from build123d import *

# Parameters (mm, degrees)
BOSS_EXTRUDE1_START = -85
SKETCH1_W           = 80
SKETCH1_H           = 12
BOSS_EXTRUDE1_DEPTH = 170
BOSS_EXTRUDE2_START = -83
SKETCH2_W           = 76
SKETCH2_H           = 14
BOSS_EXTRUDE2_DEPTH = 166
BOSS_EXTRUDE3_START = -82.6
SKETCH3_W           = 75.2
SKETCH3_H           = 16.5
BOSS_EXTRUDE3_DEPTH = 165.2
BOSS_EXTRUDE4_START = -80.6
SKETCH4_W           = 71.2
SKETCH4_H           = 17
BOSS_EXTRUDE4_DEPTH = 161.2
BOSS_EXTRUDE5_START = 50
SKETCH5_W           = 30
SKETCH5_H           = 10
BOSS_EXTRUDE5_DEPTH = 24
BOSS_EXTRUDE6_START = -74
SKETCH6_W           = 8
SKETCH6_H           = 10
BOSS_EXTRUDE6_DEPTH = 8
BOSS_EXTRUDE7_START = -45
SKETCH7_R           = 1.1
BOSS_EXTRUDE7_DEPTH = 90
BOSS_EXTRUDE8_START = -45
SKETCH8_R           = 1.1
BOSS_EXTRUDE8_DEPTH = 90


with BuildPart() as part:
    # Sketch1 → Boss-Extrude1 (new body)
    with BuildSketch(Plane.XY.offset(BOSS_EXTRUDE1_START)):
        with Locations((0, 40)):
            Rectangle(SKETCH1_W, SKETCH1_H)
    extrude(amount=BOSS_EXTRUDE1_DEPTH)


with BuildPart() as body_2:
    # Sketch2 → Boss-Extrude2 (new body)
    with BuildSketch(Plane.XY.offset(BOSS_EXTRUDE2_START)):
        with Locations((0, 37)):
            Rectangle(SKETCH2_W, SKETCH2_H)
    extrude(amount=BOSS_EXTRUDE2_DEPTH)


with BuildPart() as part_1:
    add(part.part)

    # Combine1: cut body 2
    add(body_2.part, mode=Mode.SUBTRACT)

    # Sketch3 → Boss-Extrude3 (add)
    with BuildSketch(Plane.XY.offset(BOSS_EXTRUDE3_START)):
        with Locations((0, 36.25)):
            Rectangle(SKETCH3_W, SKETCH3_H)
    extrude(amount=BOSS_EXTRUDE3_DEPTH)


with BuildPart() as body_2_2:
    # Sketch4 → Boss-Extrude4 (new body)
    with BuildSketch(Plane.XY.offset(BOSS_EXTRUDE4_START)):
        with Locations((0, 35.5)):
            Rectangle(SKETCH4_W, SKETCH4_H)
    extrude(amount=BOSS_EXTRUDE4_DEPTH)


with BuildPart() as part_2:
    add(part_1.part)

    # Combine2: cut body 2 2
    add(body_2_2.part, mode=Mode.SUBTRACT)


with BuildPart() as body_2_3:
    # Sketch5 → Boss-Extrude5 (new body)
    with BuildSketch(Plane.XY.offset(BOSS_EXTRUDE5_START)):
        with Locations((0, 45)):
            Rectangle(SKETCH5_W, SKETCH5_H)
    extrude(amount=BOSS_EXTRUDE5_DEPTH)


with BuildPart() as part_3:
    add(part_2.part)

    # Combine3: cut body 2 3
    add(body_2_3.part, mode=Mode.SUBTRACT)


with BuildPart() as body_2_4:
    # Sketch6 → Boss-Extrude6 (new body)
    with BuildSketch(Plane.XY.offset(BOSS_EXTRUDE6_START)):
        with Locations((0, 45)):
            Rectangle(SKETCH6_W, SKETCH6_H)
    extrude(amount=BOSS_EXTRUDE6_DEPTH)


with BuildPart() as part_4:
    add(part_3.part)

    # Combine4: cut body 2 4
    add(body_2_4.part, mode=Mode.SUBTRACT)


with BuildPart() as body_2_5:
    # Sketch7 → Boss-Extrude7 (new body)
    with BuildSketch(Plane(origin=(0, 0, 0), x_dir=(0, 0, -1), z_dir=(1, 0, 0)).offset(BOSS_EXTRUDE7_START)):
        with Locations(Location((30, 30, 0), (0, 0, 180))):
            Circle(SKETCH7_R)
    extrude(amount=BOSS_EXTRUDE7_DEPTH)


with BuildPart() as part_5:
    add(part_4.part)

    # Combine5: cut body 2 5
    add(body_2_5.part, mode=Mode.SUBTRACT)


with BuildPart() as body_2_6:
    # Sketch8 → Boss-Extrude8 (new body)
    with BuildSketch(Plane(origin=(0, 0, 0), x_dir=(0, 0, -1), z_dir=(1, 0, 0)).offset(BOSS_EXTRUDE8_START)):
        with Locations(Location((-30, 30, 0), (0, 0, 180))):
            Circle(SKETCH8_R)
    extrude(amount=BOSS_EXTRUDE8_DEPTH)


with BuildPart() as part_6:
    add(part_5.part)

    # Combine6: cut body 2 6
    add(body_2_6.part, mode=Mode.SUBTRACT)


solid = part_6.part
Source: CAD feature listing. Evaluate the final solid. Frame: model axes, mm. A direction names the side the tool comes from. Round coordinates to 2 decimals unless told otherwise and drop trailing zeros. Write each loop counter-clockwise with the first axis right and the second up, starting at its lowest first coordinate (ties: lowest second). Pieces come first, ordered by that corner, then holes. Notation, with made-up numbers: (-23.75, -25.75) - (22.25, -25.75) arc R14 ccw to (22.25, -13.75) - close; hole circle Ø2 at (87.25, 81.5). An arc over 180 degrees is marked (long way). Use CSV: the item, a comma, the result in double quotes. Start each with the question number.
(1) Cut plane B-B, the plane x = 28. Return loops of the section in (y, z).
(2) Cut plane C-C, the plane z = 33. Return loops of the section in (x, y), and give its area (3 significant figures).
(3) First-contact query: pin 1 Ø12 at (x, z) = (-2, -61.5) entering from -Y; pin 2 Ø8 at (x, y) = (17.5, 33) entering from +Z. Flat tips, straight axial feed; report the tip coordinate or a pass-through.
(4) Material intervals for probe 1 along X at (y, z) = (40, 32); probe 2 along Z at (x, y) = (-31, 41.5); probe 3 along Z at (x, y) = (36, 36), sorted ascending. Write a range as [from, to].
(5) Mould query, pull axis Z, two halves, no side actions, for faces 3 (the face through (-1, 36, 82.6)), 4 (the face through (-1, 40, 85)), 5 (the face through (36, 28, 0)). Classes: pulls with the +Z half, pulls with the -Z half, needs draft (parallel to the pull), parting line crosses it, or undercut.
(6) Cut plane A-A, the plane y = 41.5. Return loops of the section in (x, z), and give its area (3 significant figures).
(7) Set-up query: faces 1 (the face through (0, 36, 80.6)), 2 (the face through (-40, 40, -1)). Return all of +Z, -Z, +X, -X, +Y, -Y with unobstructed straight access to the full face (end or side cutting, diameter ignored); none if empty.
Geometry says:
1,outline,"(28, -82.6) - (44, -82.6) - (44, -83) - (34, -83) - (34, -85) - (46, -85) - (46, 85) - (34, 85) - (34, 83) - (44, 83) - (44, 82.6) - (28, 82.6) - (28, 80.6) - (44, 80.6) - (44, -80.6) - (28, -80.6) - close"
2,outline,"(-40, 34) - (-38, 34) - (-38, 44) - (-37.6, 44) - (-37.6, 28) - (-35.6, 28) - (-35.6, 44) - (35.6, 44) - (35.6, 28) - (37.6, 28) - (37.6, 44) - (38, 44) - (38, 34) - (40, 34) - (40, 46) - (-40, 46) - close"
2,area,"264 mm²"
3,pin 1,"y = 44"
3,pin 2,"z = 85"
4,probe 1,"[-40, -38], [-37.6, -35.6], [35.6, 37.6], [38, 40]"
4,probe 2,"[-85, -83], [-82.6, -80.6], [80.6, 82.6], [83, 85]"
4,probe 3,"[-85, -83], [-82.6, 82.6], [83, 85]"
5,face 3,"undercut"
5,face 4,"pulls with the +Z half"
5,face 5,"needs draft"
6,outline,"(-40, -85) - (40, -85) - (40, 85) - (-40, 85) - close; (-37.6, -82.6) - (37.6, -82.6) - (37.6, 82.6) - (-37.6, 82.6) - close; hole (-38, -83) - (38, -83) - (38, 83) - (-38, 83) - close; hole (-35.6, -80.6) - (35.6, -80.6) - (35.6, 80.6) - (-35.6, 80.6) - close"
6,area,"1,930 mm²"
7,face 1,"-Y"
7,face 2,"+Z, -Z, -X, +Y, -Y"
